Input: part model. Units: mm. Frame: model coordinates. Face numbers are marked on the shaded views. A direction names the side the tool comes from. Coordinates: 2 decimals unless noted, no trailing zeros. Loops run counter-clockwise (first coordinate to the right, second up) from the corner with the lowest first, then second, coordinate; pieces in that order, holes last.
(1) Set-up query: the marked faces 1, 2, 3, 4 and 5. Return all of +Z, -Z, +X, -X, +Y, -Y with unobstructed straight access to the full face (end or side cutting, diameter ignored); none if empty.
(2) Contact query for flat-ended pins moving along their axis: P1, Ø13.5, axis at x = 31.82, y = 31.82, coming from the +Z side; P2, Ø9, axis at x = -5, z = 35.5, coming from the -Y side; P3, Ø3, axis at y = -29, z = 21, coming from the -X side; P4, Ø2, axis at y = -16.5, z = 16, coming from the -X side. Output: stop coordinate, or through.
(3) Section C-C, the plane y = 0. Return loops of the section in (x, z).
(4) Section A-A, the plane z = 35.5. Return loops of the section in (x, y), then the cut area to 3 significant figures.
(5) Mould query, pull axis Y, two halves, no side actions, for the marked faces 6, 7, 8 and 9. Classes: released by +Y, released by -Y, zero draft, split by the parting line, or undercut.
(6) Section D-D, the plane z = 4.5. Return loops of the section in (x, y).
(7) Line query: L1, parallel to Y at x = 0, z = 17.5; L2, parallel to X at y = -27, z = 5; L3, parallel to X at y = -34, z = 6. Output: solid intervals per line, ascending.
(8) Section B-B, the plane x = 0. Return loops of the section in (y, z), then the cut area to 3 significant figures.
```python
from build123d import *

# Parameters (mm, degrees)
SKETCH_1_R          = 21.25
SKETCH_1_R_2        = 7.5
EXTRUDE_1_DEPTH     = 13
SKETCH_2_R          = 21.25
EXTRUDE_4_DEPTH     = 25
CUT_EXTRUDE_START   = -8
CUT_EXTRUDE_4_DEPTH = 8
FILLET_5_R          = 2
FILLET_6_R          = 5
CHAMFER_1_SIZE      = 1


with BuildPart() as part:
    # Эскиз1 → Бобышка-Вытянуть1 (new body)
    with BuildSketch(Plane.XY):
        with BuildLine():
            Line((-18.069008367, 40), (18.069008367, 40))
            ThreePointArc((18.069008367, 40), (36.061694556, 47.247260365), (47.819805153, 31.819805153))
            Line((47.819805153, 31.819805153), (47.819805153, -31.819805153))
            ThreePointArc((47.819805153, -31.819805153), (36.061694556, -47.247260365), (18.069008367, -40))
            Line((18.069008367, -40), (-18.069008367, -40))
            ThreePointArc((-18.069008367, -40), (-36.061694556, -47.247260365), (-47.819805153, -31.819805153))
            Line((-47.819805153, -31.819805153), (-47.819805153, 31.819805153))
            ThreePointArc((-47.819805153, 31.819805153), (-36.061694556, 47.247260365), (-18.069008367, 40))
        make_face()
        with Locations(Location((0, 0, 0), (0, 0, 180))):
            Circle(SKETCH_1_R, mode=Mode.SUBTRACT)
        with Locations(Location((-31.819805153, 31.819805153, 0), (0, 0, 180))):
            Circle(SKETCH_1_R_2, mode=Mode.SUBTRACT)
        with Locations(Location((31.819805153, 31.819805153, 0), (0, 0, 180))):
            Circle(SKETCH_1_R_2, mode=Mode.SUBTRACT)
        with Locations(Location((31.819805153, -31.819805153, 0), (0, 0, 180))):
            Circle(SKETCH_1_R_2, mode=Mode.SUBTRACT)
        with Locations(Location((-31.819805153, -31.819805153, 0), (0, 0, 180))):
            Circle(SKETCH_1_R_2, mode=Mode.SUBTRACT)
    extrude(amount=EXTRUDE_1_DEPTH)

    # Эскиз2 → Бобышка-Вытянуть4 (add)
    with BuildSketch(Plane.XY.offset(13)):
        with BuildLine():
            Line((8, -30), (-8, -30))
            ThreePointArc((-8, -30), (-11.535533906, -28.535533906), (-13, -25))
            Line((-13, -25), (-13, -24.718414189))
            ThreePointArc((-13, -24.718414189), (-13.459755187, -22.856515516), (-14.733333333, -21.42262563))
            ThreePointArc((-14.733333333, -21.42262563), (-26, 0), (-14.733333333, 21.42262563))
            ThreePointArc((-14.733333333, 21.42262563), (-13.459755187, 22.856515516), (-13, 24.718414189))
            Line((-13, 24.718414189), (-13, 25))
            ThreePointArc((-13, 25), (-11.535533906, 28.535533906), (-8, 30))
            Line((-8, 30), (8, 30))
            ThreePointArc((8, 30), (11.535533906, 28.535533906), (13, 25))
            Line((13, 25), (13, 24.718414189))
            ThreePointArc((13, 24.718414189), (13.459755187, 22.856515516), (14.733333333, 21.42262563))
            ThreePointArc((14.733333333, 21.42262563), (26, 0), (14.733333333, -21.42262563))
            ThreePointArc((14.733333333, -21.42262563), (13.459755187, -22.856515516), (13, -24.718414189))
            Line((13, -24.718414189), (13, -25))
            ThreePointArc((13, -25), (11.535533906, -28.535533906), (8, -30))
        make_face()
        with Locations(Location((0, 0, 0), (0, 0, 180))):
            Circle(SKETCH_2_R, mode=Mode.SUBTRACT)
    extrude(amount=EXTRUDE_4_DEPTH)

    # Эскиз3 → Вырез-Вытянуть4 (cut)
    with BuildSketch(Plane.XY.offset(38).offset(CUT_EXTRUDE_START)):
        with BuildLine():
            Line((-14.06568163, 22), (14.06568163, 22))
            ThreePointArc((14.06568163, 22), (14.383532605, 21.692840132), (14.733333333, 21.42262563))
            ThreePointArc((14.733333333, 21.42262563), (26, 0), (14.733333333, -21.42262563))
            ThreePointArc((14.733333333, -21.42262563), (14.383532605, -21.692840132), (14.06568163, -22))
            Line((14.06568163, -22), (-14.06568163, -22))
            ThreePointArc((-14.06568163, -22), (-14.383532605, -21.692840132), (-14.733333333, -21.42262563))
            ThreePointArc((-14.733333333, -21.42262563), (-26, 0), (-14.733333333, 21.42262563))
            ThreePointArc((-14.733333333, 21.42262563), (-14.383532605, 21.692840132), (-14.06568163, 22))
        make_face()
    extrude(amount=CUT_EXTRUDE_4_DEPTH, mode=Mode.SUBTRACT)

    # Скругление5
    fillet_5_edges = [part.edges().sort_by_distance(p)[0] for p in [
        (18.069008367, -40, 6.5),
        (-18.069008367, -40, 6.5),
        (-18.069008367, 40, 6.5),
        (18.069008367, 40, 6.5),
        (11.535533906, -28.535533906, 13),
        (13, -24.859207094, 13),
        (13.459755187, -22.856515516, 13),
        (26, 0, 13),
        (13.459755187, 22.856515516, 13),
        (13, 24.859207094, 13),
        (11.535533906, 28.535533906, 13),
        (0, 30, 13),
        (-11.535533906, 28.535533906, 13),
        (-13, 24.859207094, 13),
        (-13.459755187, 22.856515516, 13),
        (-26, 0, 13),
        (-13.459755187, -22.856515516, 13),
        (-13, -24.859207094, 13),
        (-11.535533906, -28.535533906, 13),
        (0, -30, 13),
    ]]
    fillet(fillet_5_edges, radius=FILLET_5_R)

    # Скругление6
    fillet_6_edges = [part.edges().sort_by_distance(p)[0] for p in [
        (0, 40, 13),
        (0, -40, 13),
        (-17.907285662, 40.230499291, 13),
        (17.907285662, 40.230499291, 13),
        (17.907285662, -40.230499291, 13),
        (-17.907285662, -40.230499291, 13),
        (47.819805153, 0, 13),
        (36.556686471, 47.102539051, 13),
        (-36.556686471, 47.102539051, 13),
        (-47.819805153, 0, 13),
        (-36.556686471, -47.102539051, 13),
        (36.556686471, -47.102539051, 13),
    ]]
    fillet(fillet_6_edges, radius=FILLET_6_R)

    # Фаска1
    chamfer_1_edges = [part.edges().sort_by_distance(p)[0] for p in [
        (-24.319805153, -31.819805153, 13),
        (39.319805153, -31.819805153, 13),
        (39.319805153, 31.819805153, 13),
        (-24.319805153, 31.819805153, 0),
        (39.319805153, 31.819805153, 0),
        (39.319805153, -31.819805153, 0),
        (-24.319805153, -31.819805153, 0),
        (-24.319805153, 31.819805153, 13),
    ]]
    chamfer(chamfer_1_edges, length=CHAMFER_1_SIZE)


solid = part.part
```
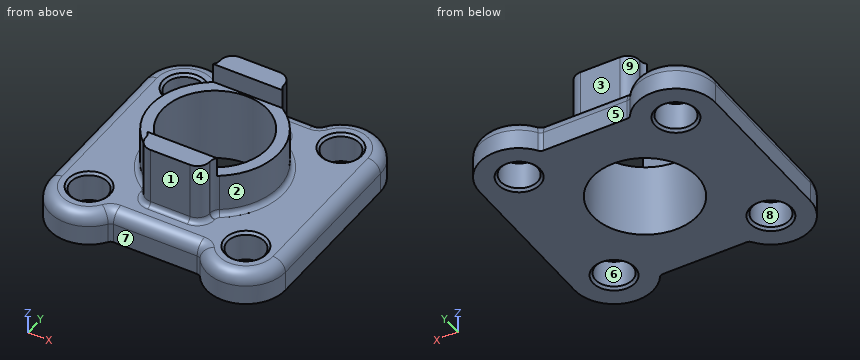
Report:
1. face 1: +Z, +X, -X, -Y
1. face 2: +Z, +X
1. face 3: +Z, +X, -X, +Y
1. face 4: +Z, +X, -Y
1. face 5: +Z, -Z, +Y
2. P1: passes through
2. P2: stops at y = -30
2. P3: stops at x = -12.33
2. P4: stops at x = -20.87
3. outline: (-47.82, 0) - (-21.25, 0) - (-21.25, 30) - (-26, 30) - (-26, 15) arc R2 cw to (-28, 13) - (-42.82, 13) arc R5 ccw to (-47.82, 8) - close; (21.25, 0) - (47.82, 0) - (47.82, 8) arc R5 ccw to (42.82, 13) - (28, 13) arc R2 cw to (26, 15) - (26, 30) - (21.25, 30) - close
4. outline: (-14.07, -22) arc R4 cw to (-13, -24.72) - (-13, -25) arc R5 ccw to (-8, -30) - (8, -30) arc R5 ccw to (13, -25) - (13, -24.72) arc R4 cw to (14.07, -22) - close; (-14.07, 22) - (14.07, 22) arc R4 cw to (13, 24.72) - (13, 25) arc R5 ccw to (8, 30) - (-8, 30) arc R5 ccw to (-13, 25) - (-13, 24.72) arc R4 cw to start
4. area: 398 mm2
5. face 6: undercut
5. face 7: released by -Y
5. face 8: undercut
5. face 9: released by +Y
6. outline: (-47.82, -31.82) arc R16 ccw to (-18.62, -40.87) arc R2 cw to (-16.98, -40) - (16.98, -40) arc R2 cw to (18.62, -40.87) arc R16 ccw to (47.82, -31.82) - (47.82, 31.82) arc R16 ccw to (18.62, 40.87) arc R2 cw to (16.98, 40) - (-16.98, 40) arc R2 cw to (-18.62, 40.87) arc R16 ccw to (-47.82, 31.82) - close; hole circle Ø15 at (-31.82, -31.82); hole circle Ø15 at (-31.82, 31.82); hole circle Ø42.5 at (0, 0); hole circle Ø15 at (31.82, -31.82); hole circle Ø15 at (31.82, 31.82)
7. L1: y = -30 to -21.25, 21.25 to 30
7. L2: x = -47.82 to -37.57, -26.07 to 26.07, 37.57 to 47.82
7. L3: x = -47.67 to -39, -24.64 to 24.64, 39 to 47.67
8. outline: (-40, 0) - (-21.25, 0) - (-21.25, 30) - (-22, 30) - (-22, 38) - (-30, 38) - (-30, 15) arc R2 cw to (-32, 13) - (-35, 13) arc R5 ccw to (-40, 8) - close; (21.25, 0) - (40, 0) - (40, 8) arc R5 ccw to (35, 13) - (32, 13) arc R2 cw to (30, 15) - (30, 38) - (22, 38) - (22, 30) - (21.25, 30) - close
8. area: 904 mm2
